Here's how the part is built. I have some questions about the finished solid (model axes, mm). A direction names the side the tool comes from. Round coordinates to 2 decimals unless told otherwise and drop trailing zeros. Loops run counter-clockwise (first coordinate to the right, second up) from the corner with the lowest first, then second, coordinate; pieces in that order, holes last. Notation, with made-up numbers: M -31.75,75 L 21.25,75 A17 ccw 21.25,83 Z; hole C 53,52 d1. An arc over 180 degrees is marked long. Use a Markdown table: item, result.
```python
from build123d import *

# Parameters (mm, degrees)
BOSS_EXTRUDE1_DEPTH = 2


with BuildPart() as part:
    # Sketch1 → Boss-Extrude1 (new body)
    with BuildSketch(Plane.XY):
        with BuildLine():
            Line((-26.329238207, -11.829238207), (-26.329238207, -10.829238207))
            ThreePointArc((-26.329238207, -10.829238207), (-26.036344989, -10.122131426), (-25.329238207, -9.829238207))
            Line((-25.329238207, -9.829238207), (-7.329238207, -9.829238207))
            ThreePointArc((-7.329238207, -9.829238207), (-6.622131426, -10.122131426), (-6.329238207, -10.829238207))
            Line((-6.329238207, -10.829238207), (-6.329238207, -11.829238207))
            Line((-6.329238207, -11.829238207), (16.170761793, -11.829238207))
            Line((16.170761793, -11.829238207), (16.170761793, -20.079238207))
            Line((16.170761793, -20.079238207), (6.170761793, -20.079238207))
            Line((6.170761793, -20.079238207), (6.170761793, -20.329238207))
            Line((6.170761793, -20.329238207), (-12.829238207, -20.329238207))
            Line((-12.829238207, -20.329238207), (-14.329238207, -22.329238207))
            Line((-14.329238207, -22.329238207), (-16.329238207, -22.329238207))
            Line((-16.329238207, -22.329238207), (-18.329238207, -22.329238207))
            Line((-18.329238207, -22.329238207), (-19.829238207, -20.329238207))
            Line((-19.829238207, -20.329238207), (-38.829238207, -20.329238207))
            Line((-38.829238207, -20.329238207), (-38.829238207, -20.079238207))
            Line((-38.829238207, -20.079238207), (-48.829238207, -20.079238207))
            Line((-48.829238207, -20.079238207), (-48.829238207, -11.829238207))
            Line((-48.829238207, -11.829238207), (-26.329238207, -11.829238207))
        make_face()
    extrude(amount=BOSS_EXTRUDE1_DEPTH)


solid = part.part
```
Q1. I need wall thicknesses on line 1 (Y direction, x = -45.5, z = 1.2); line 2 (Y direction, x = -33.5, z = 0.1); line 3 (X direction, y = -11.5, z = 0.4). Which ranges of each line are inside material? Lowest first, please. Write a range as from..to.
Return value:
| item | result |
|---|---|
| line 1 | y = -20.08..-11.83 |
| line 2 | y = -20.33..-11.83 |
| line 3 | x = -26.33..-6.33 |
Q2. Imagine slicing it at B-B, the plane x = -33.5. Please give me the cut outline in (y, z).
Return value:
| item | result |
|---|---|
| outline | M -20.33,0 L -11.83,0 L -11.83,2 L -20.33,2 Z |
Q3. For faces 1 (the flat face through (11, -20.079, 1)), 2 (the flat face through (-48.829, -16, 1)), 3 (the flat face through (-29, -20.329, 1)), 4 (the flat face through (5, -11.829, 1)), 5 (the flat face through (-26.329, -11, 1)), which set-ups out of +Z, -Z, +X, -X, +Y, -Y let a thin tool reach every point of the face, with its end or its side?
Return value:
| item | result |
|---|---|
| face 1 | +Z, -Z, +X, -Y |
| face 2 | +Z, -Z, -X, +Y, -Y |
| face 3 | +Z, -Z, -X, -Y |
| face 4 | +Z, -Z, +X, +Y |
| face 5 | +Z, -Z, -X, +Y |
Q4. Will these pins go through, and if not, where does the flat tip stop? P1, Ø0.6, axis at x = -46, z = 1.5, coming from the -Y side; P2, Ø6, axis at x = -31, y = -20.5, coming from the -Z side; P3, Ø0.8, axis at y = -11, z = 1.5, coming from the -X side; P4, Ø0.6, axis at x = 4, z = 0.5, coming from the +Y side.
Return value:
| item | result |
|---|---|
| P1 | stops at y = -20.08 |
| P2 | stops at z = 0 |
| P3 | stops at x = -26.33 |
| P4 | stops at y = -11.83 |
Q5. Imagine slicing it at A-A, the plane z = 1.05. Please give me the cut outline in (x, y), then the cut area to 3 significant figures.
Return value:
| item | result |
|---|---|
| outline | M -48.83,-20.08 L -38.83,-20.08 L -38.83,-20.33 L -19.83,-20.33 L -18.33,-22.33 L -14.33,-22.33 L -12.83,-20.33 L 6.17,-20.33 L 6.17,-20.08 L 16.17,-20.08 L 16.17,-11.83 L -6.33,-11.83 L -6.33,-10.83 A1 ccw -7.33,-9.83 L -25.33,-9.83 A1 ccw -26.33,-10.83 L -26.33,-11.83 L -48.83,-11.83 Z |
| area | 598 mm^2 |
Q6. Imagine slicing it at C-C, the plane x = -43.5. Please give me the cut outline in (y, z), then the cut area to 3 significant figures.
Return value:
| item | result |
|---|---|
| outline | M -20.08,0 L -11.83,0 L -11.83,2 L -20.08,2 Z |
| area | 16.5 mm^2 |
